from build123d import *

# Parameters (mm, degrees)
SKETCH2_R           = 72.5
SKETCH2_R_2         = 1.4732
BOSS_EXTRUDE3_DEPTH = 0.254


with BuildPart() as part:
    # Sketch2 → Boss-Extrude3 (new body)
    with BuildSketch(Plane.XY):
        Circle(SKETCH2_R)
        with Locations((56.291651246, -32.5)):
            Circle(SKETCH2_R_2, mode=Mode.SUBTRACT)
        with Locations((0, -65)):
            Circle(SKETCH2_R_2, mode=Mode.SUBTRACT)
        with Locations((-56.291651246, -32.5)):
            Circle(SKETCH2_R_2, mode=Mode.SUBTRACT)
        with Locations((-56.291651246, 32.5)):
            Circle(SKETCH2_R_2, mode=Mode.SUBTRACT)
        with Locations((0, 65)):
            Circle(SKETCH2_R_2, mode=Mode.SUBTRACT)
        with Locations((56.291651246, 32.5)):
            Circle(SKETCH2_R_2, mode=Mode.SUBTRACT)
        Polygon((-0.5, 50), (-0.5, 0.5), (-50, 0.5), (-50, -0.5), (-0.5, -0.5), (-0.5, -50), (0.5, -50), (0.5, -0.5), (50, -0.5), (50, 0.5), (0.5, 0.5), (0.5, 50), align=None, mode=Mode.SUBTRACT)
    extrude(amount=BOSS_EXTRUDE3_DEPTH)


solid = part.part
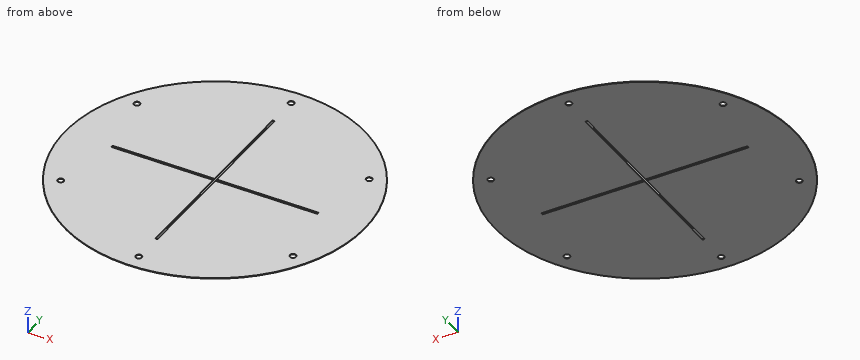
The listing builds one solid part. Answer for the finished solid, in the listing's coordinates (mm). Round coordinates to 2 decimals unless told otherwise and drop trailing zeros. Order: outer loops, then holes, each group sorted by start corner. A loop starts at its lowest first (then second) coordinate and runs counter-clockwise, first axis right, second up. Notation, with made-up numbers: (39, 80.5) - (70, 80.5) arc R18 ccw to (70, 94.5) - close; hole circle Ø2 at (-29, 32). An arc over 180 degrees is marked (long way). Write item = value, one per line. Start each with the question number.
1) Section B-B, the plane x = 19.5 is taken. Write down the section's boundary in (y, z), plus the area to 3 significant figures.
2) Section A-A, the plane z = 0.05 is taken. Write down the section's boundary in (x, y).
3) Section D-D, the plane y = -61.5 is taken. Write down the section's boundary in (x, z), plus the area to 3 significant figures.
4) Given pin 1 (4 mm diameter, centred on x = -56.29, y = 32.5, fed in from +Z); pin 2 (2.5 mm diameter, centred on x = 56.29, y = 32.5, fed in from +Z), each flat-ended and moving along its own axis, determine where each tip first touches the part or whether it passes through.
5) Section C-C, the plane y = -14.5 is taken. Write down the section's boundary in (x, z).
6) Straight lines are drawn through the part: L1, parallel to Y at x = 0, z = 0.1; L2, parallel to Y at x = 9, z = 0.1; L3, parallel to Y at x = -16, z = 0.1. For each, find the intervals that lie inside material, in ascending order.
Results list:
q1.outline = (-69.83, 0) - (-0.5, 0) - (-0.5, 0.25) - (-69.83, 0.25) - close; (0.5, 0) - (69.83, 0) - (69.83, 0.25) - (0.5, 0.25) - close
q1.area = 35.2 mm^2
q2.outline = circle Ø145 at (0, 0); hole circle Ø2.95 at (-56.29, -32.5); hole circle Ø2.95 at (-56.29, 32.5); hole (-50, -0.5) - (-0.5, -0.5) - (-0.5, -50) - (0.5, -50) - (0.5, -0.5) - (50, -0.5) - (50, 0.5) - (0.5, 0.5) - (0.5, 50) - (-0.5, 50) - (-0.5, 0.5) - (-50, 0.5) - close; hole circle Ø2.95 at (0, -65); hole circle Ø2.95 at (0, 65); hole circle Ø2.95 at (56.29, -32.5); hole circle Ø2.95 at (56.29, 32.5)
q3.outline = (-38.39, 0) - (38.39, 0) - (38.39, 0.25) - (-38.39, 0.25) - close
q3.area = 19.5 mm^2
q4.pin_1 = 0.25
q4.pin_2 = through
q5.outline = (-71.04, 0) - (-0.5, 0) - (-0.5, 0.25) - (-71.04, 0.25) - close; (0.5, 0) - (71.04, 0) - (71.04, 0.25) - (0.5, 0.25) - close
q6.L1 = -72.5 to -66.47, -63.53 to -50, 50 to 63.53, 66.47 to 72.5
q6.L2 = -71.94 to -0.5, 0.5 to 71.94
q6.L3 = -70.71 to -0.5, 0.5 to 70.71
